For this review, take the finished solid that the model builds, in its own axes (mm). A direction names the side the tool comes from. Round coordinates to 2 decimals unless told otherwise and drop trailing zeros. Loops run counter-clockwise (first coordinate to the right, second up) from the corner with the lowest first, then second, coordinate; pieces in that order, holes last.
1. Consider section A-A on x = -5.08. State the section outline as (y, z) points.
2. Clearance check with a flat-ended pin moving along its axis: pin 1 Ø0.8 at (y, z) = (0.5, -55.5) entering from +X. State where the tip first meets the part, or that it passes through.
3. Draft analysis for pull direction X (two halves, no side actions). For faces 3 (the cylindrical face through (-0.91, 0.8, -93.03)), 4 (the cylindrical face through (-93.1, 0.8, -84.8)), 5 (the cylindrical face through (-24.145, 0.783, -16.758)), state which applies: released by +X, released by -X, zero draft, split by the parting line, or undercut.
4. To check wall thickness, follow line 1 along X through (y, z) = (0.6, -88.9); line 2 along X through (y, z) = (0.35, -78.5); line 3 along Z through (x, y) = (-8.5, 0.75). State the ranges of each line that lie inside material, in increasing order.
5. Consider section D-D on z = -5.08. State the section outline as (x, y) points.
6. Consider section B-B on z = -78.74. State the section outline as (x, y) points, then the cut area to 3 significant figures.
7. Consider section C-C on y = 0.4. State how many separate pieces and enclosed holes the cut face has, then the cut area to 3 significant figures.
8. Tool access review of faces 1 (the cylindrical face through (-4.852, 0.783, -90.635)), 2 (the cylindrical face through (-11.75, 0.8, -82.91)): name each direction out of +Z, -Z, +X, -X, +Y, -Y from which nothing blocks a thin tool from reaching the whole face with its end or side.
Autodesk Inventor part; units mm, degrees
ref_plane "YZ Plane" through (0, 0, 0) normal (1, 0, 0) x (0, 1, 0)
ref_plane "XZ Plane" through (0, 0, 0) normal (0, 1, 0) x (-1, 0, 0)
ref_plane "XY Plane" through (0, 0, 0) normal (0, 0, 1) x (1, 0, 0)
sketch "Sketch1" plane through (0, 0, 0) normal (0, 1, 0) x (-1, 0, 0)
  line L0 (0, 0) -> (93.98, 0)
  line L1 (93.98, -93.98) -> (0, -93.98)
  circle A0 centre (88.9, -5.08) radius 1.75
  circle A1 centre (5.08, -5.08) radius 1.75
  circle A2 centre (5.08, -88.9) radius 1.75
  circle A3 centre (88.9, -88.9) radius 1.75
  circle A4 centre (23.1775, -78.74) radius 1.8
  circle A5 centre (23.1775, -78.74) radius 1.8
  circle A6 centre (70.8025, -78.74) radius 1.8
  circle A7 centre (70.8025, -78.74) radius 1.8
  circle A8 centre (70.8025, -15.24) radius 1.8
  circle A9 centre (70.8025, -15.24) radius 1.8
  circle A10 centre (23.1775, -15.24) radius 1.8
  circle A11 centre (23.1775, -15.24) radius 1.8
  line L2 (93.98, 0) -> (93.98, -10.16)
  line L3 (93.98, -10.16) -> (81.28, -10.16)
  line L4 (93.98, -93.98) -> (93.98, -83.82)
  line L5 (93.98, -83.82) -> (81.28, -83.82)
  line L6 (81.28, -83.82) -> (81.28, -10.16)
  line L7 (0, -10.16) -> (12.7, -10.16)
  line L8 (0, -83.82) -> (12.7, -83.82)
  line L9 (12.7, -83.82) -> (12.7, -10.16)
  line L10 (93.98, 0) -> (93.98, -10.16)
  line L11 (93.98, -83.82) -> (93.98, -93.98)
  line L12 (0, -93.98) -> (0, -83.82)
  line L13 (0, -10.16) -> (0, 0)
extrude "Extrusion1" add sketch "Sketch1" along normal blind 1.5875
fillet "Fillet1" radius 3.175 12 edges at (0, 0.7937, 0) (0, 0.7937, -10.16) (-12.7, 0.7937, -10.16) (-12.7, 0.7937, -83.82) (0, 0.7937, -83.82) (0, 0.7937, -93.98) (-93.98, 0.7937, 0) (-93.98, 0.7937, -10.16) (-81.28, 0.7937, -10.16) (-81.28, 0.7937, -83.82) (-93.98, 0.7937, -83.82) (-93.98, 0.7937, -93.98)
properties part number "ethernetPlate"
Resolved:
1. outline: (0, -93.98) - (1.59, -93.98) - (1.59, -90.65) - (0, -90.65) - close; (0, -87.15) - (1.59, -87.15) - (1.59, -83.82) - (0, -83.82) - close; (0, -10.16) - (1.59, -10.16) - (1.59, -6.83) - (0, -6.83) - close; (0, -3.33) - (1.59, -3.33) - (1.59, 0) - (0, 0) - close
2. pin 1: stops at x = -12.7
3. face 3: released by +X
3. face 4: released by -X
3. face 5: undercut
4. line 1: x = -93.98 to -90.65, -87.15 to -6.83, -3.33 to 0
4. line 2: x = -81.28 to -72.59, -69.02 to -24.96, -21.39 to -12.7
4. line 3: z = -93.98 to -83.82, -10.16 to 0
5. outline: (-93.98, 0) - (-90.65, 0) - (-90.65, 1.59) - (-93.98, 1.59) - close; (-87.15, 0) - (-6.83, 0) - (-6.83, 1.59) - (-87.15, 1.59) - close; (-3.33, 0) - (0, 0) - (0, 1.59) - (-3.33, 1.59) - close
6. outline: (-81.28, 0) - (-72.6, 0) - (-72.6, 1.59) - (-81.28, 1.59) - close; (-69, 0) - (-24.98, 0) - (-24.98, 1.59) - (-69, 1.59) - close; (-21.38, 0) - (-12.7, 0) - (-12.7, 1.59) - (-21.38, 1.59) - close
6. area: 97.4 mm2
7. separate pieces: 1
7. enclosed holes: 8
7. area: 6,870 mm2
8. face 1: +Y, -Y
8. face 2: +X, +Y, -Y
